Could you check a few things on this drawing? It's one solid part, dimensions in mm from its lowest x, y, z. A direction names the side the tool comes from. Give positions to 0.01 mm unless a question says otherwise; leave off trailing zeros. Write each loop counter-clockwise with the first axis right and the second up, starting at its lowest first coordinate (ties: lowest second). Pieces come first, ordered by that corner, then holes. Notation, with made-up numbers: (67.5, -29.5) -> (81.5, -29.5) arc R19 ccw to (81.5, -1.5) -> close; hole circle Ø7 at (46, 78). An arc over 180 degrees is marked (long way). Answer as CSV lines item,"result". Start each with the question number.
1. If we section it at A-A on z = 6: Write out the boundary of the cut face in (x, y).
2. If we section it at B-B on x = 6: Write out the boundary of the cut face in (y, z).
3. I need wall thicknesses on line 1 (Y direction, x = 0.5, z = 5.25); line 2 (Z direction, x = 6, y = 15); line 3 (Z direction, x = 6, y = 10). Which ranges of each line are inside material? Lowest first, please. Write a range as [from, to].
4. If we section it at D-D on x = 2: Write out the boundary of the cut face in (y, z) (3 decimals).
5. If we mould it in two halves opening along Y, with no side actions, what happens to the marked faces 1, 2 and 3? For each: pulls with the +Y half, pulls with the -Y half, needs draft (parallel to the pull), parting line crosses it, or undercut.
6. I'm going to push flat-ended pins straight in: P1, Ø2, axis at x = 10.5, y = 14, coming from the -Z side; P2, Ø1, axis at x = 11, y = 14, coming from the -Z side; P3, Ø5, axis at x = 9, y = 10.5, coming from the +Z side; P4, Ø4, axis at x = 6, z = 6, coming from the -Y side. Where does each tip first touch, or does it pass through?
7. If we section it at C-C on y = 13: Write out the boundary of the cut face in (x, z), plus the area to 3 significant figures.
8. On a 3-axis mill with a long thin cutter (end or side, diameter ignored), from which of +Z, -Z, +X, -X, +Y, -Y can I reach the whole of each face in a straight line? I mean the marked faces 4 and 5. Say none if no direction works.
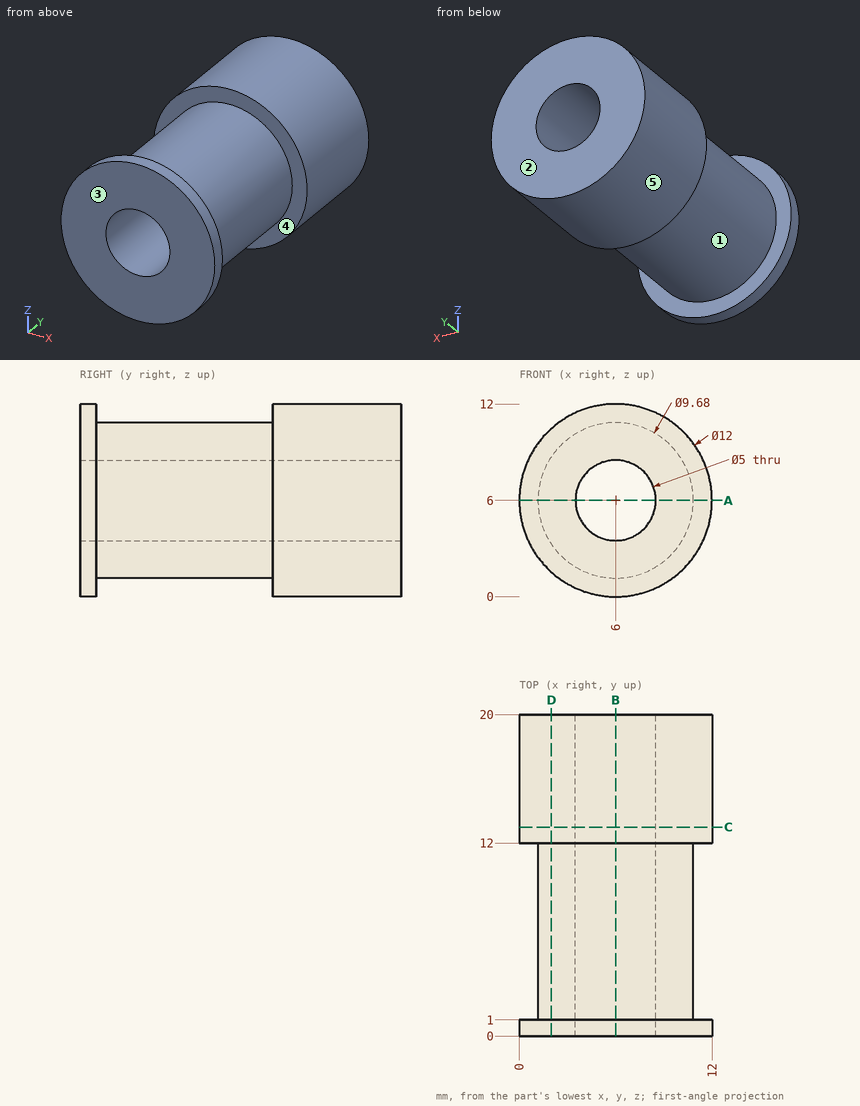
Computed values:
1,outline,"(0, 0) -> (3.5, 0) -> (3.5, 20) -> (0, 20) -> (0, 12) -> (1.16, 12) -> (1.16, 1) -> (0, 1) -> close; (8.5, 0) -> (12, 0) -> (12, 1) -> (10.84, 1) -> (10.84, 12) -> (12, 12) -> (12, 20) -> (8.5, 20) -> close"
2,outline,"(0, 0) -> (1, 0) -> (1, 1.16) -> (12, 1.16) -> (12, 0) -> (20, 0) -> (20, 3.5) -> (0, 3.5) -> close; (0, 8.5) -> (20, 8.5) -> (20, 12) -> (12, 12) -> (12, 10.84) -> (1, 10.84) -> (1, 12) -> (0, 12) -> close"
3,line 1,"y = [0, 1], [12, 20]"
3,line 2,"z = [0, 3.5], [8.5, 12]"
3,line 3,"z = [1.16, 3.5], [8.5, 10.84]"
4,outline,"(0, 1.528) -> (1, 1.528) -> (1, 3.275) -> (12, 3.275) -> (12, 1.528) -> (20, 1.528) -> (20, 10.472) -> (12, 10.472) -> (12, 8.725) -> (1, 8.725) -> (1, 10.472) -> (0, 10.472) -> close"
5,face 1,"undercut"
5,face 2,"pulls with the +Y half"
5,face 3,"pulls with the -Y half"
6,P1,"stops at z = 1.13"
6,P2,"stops at z = 2.03"
6,P3,"stops at z = 11.92"
6,P4,"passes through"
7,outline,"circle Ø12 at (6, 6); hole circle Ø5 at (6, 6)"
7,area,"93.5 mm2"
8,face 4,"none"
8,face 5,"+Y, -Y"
